Autodesk Inventor part; units mm, degrees
ref_plane "YZ Plane" through (0, 0, 0) normal (1, 0, 0) x (0, 1, 0)
ref_plane "XZ Plane" through (0, 0, 0) normal (0, 1, 0) x (-1, 0, 0)
ref_plane "XY Plane" through (0, 0, 0) normal (0, 0, 1) x (1, 0, 0)
sketch "Sketch1" plane through (0, 0, 0) normal (0, 1, 0) x (-1, 0, 0)
  line L0 (0, -2.8868) -> (-2.5, -1.4434)
  line L1 (-2.5, -1.4434) -> (-2.5, 1.4434)
  line L2 (-2.5, 1.4434) -> (0, 2.8868)
  line L3 (0, 2.8868) -> (2.5, 1.4434)
  line L4 (2.5, 1.4434) -> (2.5, -1.4434)
  line L5 (2.5, -1.4434) -> (0, -2.8868)
  point P0 (0, 0)
  point P1 (0, 0)
  dimension "d0" = 5
extrude "Extrusion1" add sketch "Sketch1" along normal blind 6
sketch "Sketch2" plane through (0, 6, 0) normal (0, 1, 0) x (1, 0, 0)
  point P0 (0, 0)
  point P1 (0, 0)
hole "Hole1" at (0, 6, 0) direction (0, -1, 0) diameter 3 end through all
sketch "Sketch3" plane through (0, 0, 0) normal (0, 0, 1) x (1, 0, 0)
  line L0 (0, 6) -> (2.5, 6)
  line L1 (2.5, 6) -> (4.5, 6)
  line L2 (2.5, 6) -> (4.5, 4.8453)
  line L3 (2.5, 6) -> (4.8094, 6) construction
  line L4 (4.5, 4.8453) -> (4.5, 6)
  line L5 (2.5, 0) -> (2.5, 6)
  line L6 (2.5, 0) -> (4.5, 0)
  line L7 (2.5, 0) -> (4.5, 1.1547)
  line L8 (2.5, 0) -> (4.8094, 0) construction
  line L9 (4.5, 1.1547) -> (4.5, 0)
  line L10 (0, -1.6) -> (0, 9.6)
  point P0 (0, 0)
  dimension "d10" = 30
  dimension "d11" = 2
  dimension "d12" = 30
revolve "Revolution1" cut sketch "Sketch3" angle 360 about axis through (0, -10, 0) along (0, 1, 0)
properties part number "M3_H8.0mm_board_spacer" material "Nickel-Copper Alloy 400"
Geometry: final body of the model. Coordinates: model frame, mm. Round coordinates to 2 decimals unless told otherwise and drop trailing zeros. Order: outer loops, then holes, each group sorted by start corner. A loop starts at its lowest first (then second) coordinate and runs counter-clockwise, first axis right, second up. Notation, with made-up numbers: (14.5, -33) -> (51.5, -33) arc R7 cw to (51.5, -26) -> close; hole circle Ø10 at (89.25, -37). An arc over 180 degrees is marked (long way). Put each result on its own line as item: value. Start each with the question number.
Q1. Section A-A on y = 3.05. Return the cut outline in (x, z), and give its area (3 significant figures).
Q2. Line query: probe 1 along X at (y, z) = (1.2, -0.4); probe 2 along X at (y, z) = (3.35, 0); probe 3 along Z at (x, y) = (0.25, 2.05). Output: solid intervals per line, ascending.
Q3. Pull-direction query (X, two-part tool) for faces 1 (the cylindrical face through (-0.07, 2.96, -1.5)), 2 (the conical face through (-0.058, 0.088, 2.652)), 3 (the flat face through (2.5, 3, 0)), 4 (the flat face through (-2.5, 3, 0)); classes: +X half, -X half, draft (parallel to the pull), parting line (faces both ways), or undercut.
Q4. First-contact query: pin 1 (1.5 mm diameter, centred on x = -0.5, y = 4, fed in from -Z); pin 2 (1 mm diameter, centred on x = -0.5, z = 0.5, fed in from +Y). Flat tips, straight axial feed; report the tip coordinate or a pass-through.
Ans:
1. outline: (-2.5, -1.44) -> (0, -2.89) -> (2.5, -1.44) -> (2.5, 1.44) -> (0, 2.89) -> (-2.5, 1.44) -> close; hole circle Ø3 at (0, 0)
1. area: 14.6 mm2
2. probe 1: x = -2.5 to -1.45, 1.45 to 2.5
2. probe 2: x = -2.5 to -1.5, 1.5 to 2.5
2. probe 3: z = -2.74 to -1.48, 1.48 to 2.74
3. face 1: undercut
3. face 2: parting line
3. face 3: +X half
3. face 4: -X half
4. pin 1: stops at z = -2.89
4. pin 2: passes through
